Read the model definition and answer for the solid it produces. Units are mm, in the model's axes. Face numbers are marked on the shaded views. Coordinates: 2 decimals unless noted, no trailing zeros. Write each loop counter-clockwise with the first axis right and the second up, starting at its lowest first coordinate (ties: lowest second). Pieces come first, ordered by that corner, then holes. Notation, with made-up numbers: (-14, 80) - (44, 80) arc R22 ccw to (44, 117) - close; hole circle Ø9 at (-30, 73.5). An arc over 180 degrees is marked (long way). Return JSON: item names as keys, results as strings.
```python
from build123d import *

# Parameters (mm, degrees)
SKIZZE1_R                                            = 2
AUFSATZ_LINEAR_AUSTRAGEN1_DEPTH                      = 5.5
VERRUNDUNG1_R                                        = 4
M3_GEWINDEBOHRUNG1_D                                 = 2.5
STIRNSENKUNG_F_R_M3_ZYLINDERSCHRAUBE_MIT_D           = 3.2
STIRNSENKUNG_F_R_M3_ZYLINDERSCHRAUBE_MIT_CBORE_D     = 6.5
STIRNSENKUNG_F_R_M3_ZYLINDERSCHRAUBE_MIT_CBORE_DEPTH = 10


with BuildPart() as part:
    # Skizze1 → Aufsatz-Linear austragen1 (new body, symmetric)
    with BuildSketch(Plane(origin=(0, 0, 0), x_dir=(1, 0, 0), z_dir=(0, 1, 0))):
        with BuildLine():
            Line((-80, 4), (-45, 4))
            Line((-45, 4), (-41, 4))
            Line((-41, 4), (-41, -10))
            Line((-41, -10), (0, -10))
            Line((0, -10), (0, -20))
            ThreePointArc((0, -20), (-36.187419929, -16.834010994), (-71.275303416, -7.43224095))
            Line((-71.275303416, -7.43224095), (-81.368080573, -3.758770483))
            ThreePointArc((-81.368080573, -3.758770483), (-83.939231012, 0.694592711), (-80, 4))
        make_face()
        with Locations((-80, 0)):
            Circle(SKIZZE1_R, mode=Mode.SUBTRACT)
    extrude(amount=AUFSATZ_LINEAR_AUSTRAGEN1_DEPTH, both=True)

    # Verrundung1
    verrundung1_edges = [part.edges().sort_by_distance(p)[0] for p in [
        (-41, 0, 10),
    ]]
    fillet(verrundung1_edges, radius=VERRUNDUNG1_R)

    # M3 Gewindebohrung1 (through all)
    with Locations(Plane(origin=(0, 5.5, 0), x_dir=(1, 0, 0), z_dir=(0, 1, 0))):
        with Locations((-45, 0)):
            Hole(M3_GEWINDEBOHRUNG1_D / 2)

    # Spiegeln3: part across plane


with BuildPart() as part_1:
    add(part.part)
    add(part.part.mirror(Plane(origin=(0, 0, 0), x_dir=(0, 0, 1), z_dir=(1, 0, 0))))

    # Stirnsenkung für  M3 Zylinderschraube mit Schlitz/Kreuzschlitz1 (through all)
    with Locations(Plane.XY.offset(20)):
        with Locations((-45, 0), (45, 0)):
            CounterBoreHole(STIRNSENKUNG_F_R_M3_ZYLINDERSCHRAUBE_MIT_D / 2, STIRNSENKUNG_F_R_M3_ZYLINDERSCHRAUBE_MIT_CBORE_D / 2, STIRNSENKUNG_F_R_M3_ZYLINDERSCHRAUBE_MIT_CBORE_DEPTH)


solid = part_1.part
```
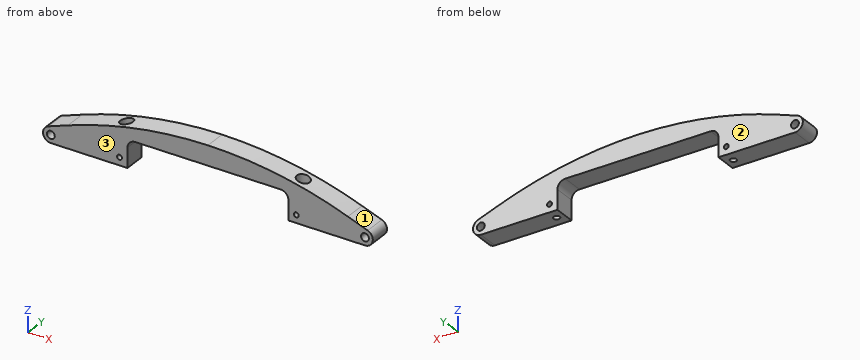
(1) Determine the mould class of the marked faces 1, 2 and 3 for opening direction Y: +Y half, -Y half, draft (parallel to the pull), parting line (faces both ways), or undercut.
Answer:
{"face 1": "draft", "face 2": "+Y half", "face 3": "-Y half"}
(2) Flat-ended cylindrical pins translate along their axes: P1, Ø5, axis at x = 15.5, y = -2, coming from the +Z side; P2, Ø1.5, axis at x = 65.5, y = 1, coming from the +Z side; P3, Ø2, axis at x = 45, z = 0, coming from the -Y side; P4, Ø1.5, axis at x = -24.5, y = -4.5, coming from the -Z side. Find the tip coordinate at first contact, or state that the pin passes through.
Answer:
{"P1": "z = 19.59", "P2": "z = 9.69", "P3": "through", "P4": "z = 10"}
(3) Straight lines are drawn through the part: line 1 (Y direction, x = -45, z = 11.4); line 2 (Z direction, x = 45, y = -3.15); line 3 (Z direction, x = -45, y = 4.3). For each, find the intervals that lie inside material, in ascending order. Write a range as from..to.
Answer:
{"line 1": "-5.5..-3.25, 3.25..5.5", "line 2": "-4..-1.25, 1.25..10", "line 3": "-4..-1.25, 1.25..15.08"}
(4) A cutting plane is placed at A-A (x = -53.5). Determine the outline of the cut face in (y, z).
Answer:
{"outline": "(-5.5, -4) - (5.5, -4) - (5.5, 13.02) - (-5.5, 13.02) - close"}
